from build123d import *

# Parameters (mm, degrees)
SCHIZZO1_R                   = 14
ESTRUSIONE_ESTRUSIONE1_DEPTH = 19.5
TAGLIO_ESTRUSIONE1_START     = -4
SCHIZZO2_R                   = 1
TAGLIO_ESTRUSIONE1_DEPTH     = 4
SCHIZZO3_R                   = 4.27486225
ESTRUSIONE_ESTRUSIONE2_DEPTH = 1.5
SCHIZZO4_R                   = 11.5
TAGLIO_ESTRUSIONE2_DEPTH     = 16.5
SCHIZZO5_R                   = 1.5
TAGLIO_ESTRUSIONE3_DEPTH     = 16.5
TAGLIO_ESTRUSIONE4_START     = -4
TAGLIO_ESTRUSIONE4_DEPTH     = 4
SCHIZZO7_R                   = 1.5
ESTRUSIONE_ESTRUSIONE3_DEPTH = 27.5
SCHIZZO8_R                   = 4
ESTRUSIONE_ESTRUSIONE4_DEPTH = 3
SCHIZZO9_W                   = 0.1
SCHIZZO9_H                   = 14.938811625
SMUSSO1_SIZE                 = 3.5
SMUSSO1_SIZE2                = 0.680331082
SMUSSO2_SIZE                 = 0.720279458
SMUSSO2_SIZE_2               = 3.5


with BuildPart() as part:
    # Schizzo1 → Estrusione-Estrusione1 (new body)
    with BuildSketch(Plane(origin=(0, 0, 0), x_dir=(1, 0, 0), z_dir=(0, 1, 0))):
        with Locations(Location((0, 0, 0), (0, 0, 270))):
            Circle(SCHIZZO1_R)
    extrude(amount=ESTRUSIONE_ESTRUSIONE1_DEPTH)

    # Schizzo2 → Taglio-Estrusione1 (cut)
    with BuildSketch(Plane(origin=(0, 19.5, 0), x_dir=(1, 0, 0), z_dir=(0, 1, 0)).offset(TAGLIO_ESTRUSIONE1_START)):
        with BuildLine():
            Line((-7.95445115, 11.520707743), (0, 4.27486225))
            Line((0, 4.27486225), (7.95445115, 11.520707743))
            ThreePointArc((7.95445115, 11.520707743), (0, 14), (-7.95445115, 11.520707743))
        make_face()
        with BuildLine():
            ThreePointArc((14, 0), (13.988608153, 0.564660915), (13.95445115, 1.128402898))
            Line((13.95445115, 1.128402898), (3.702139306, -2.137431125))
            Line((3.702139306, -2.137431125), (6, -12.649110641))
            ThreePointArc((6, -12.649110641), (11.832159566, -7.483314774), (14, 0))
        make_face()
        with BuildLine():
            Line((-3.702139306, -2.137431125), (-13.95445115, 1.128402898))
            ThreePointArc((-13.95445115, 1.128402898), (-12.124355653, -7), (-6, -12.649110641))
            Line((-6, -12.649110641), (-3.702139306, -2.137431125))
        make_face()
        with Locations(Location((0, -6, 0), (0, 0, 270))):
            Circle(SCHIZZO2_R)
        with Locations(Location((-5.196152423, 3, 0), (0, 0, 270))):
            Circle(SCHIZZO2_R)
        with Locations(Location((5.196152423, 3, 0), (0, 0, 270))):
            Circle(SCHIZZO2_R)
    extrude(amount=TAGLIO_ESTRUSIONE1_DEPTH, mode=Mode.SUBTRACT)

    # Schizzo3 → Estrusione-Estrusione2 (add)
    with BuildSketch(Plane(origin=(0, 19.5, 0), x_dir=(1, 0, 0), z_dir=(0, 1, 0))):
        with Locations(Location((0, 0, 0), (0, 0, 90))):
            Circle(SCHIZZO3_R)
    extrude(amount=ESTRUSIONE_ESTRUSIONE2_DEPTH)

    # Schizzo4 → Taglio-Estrusione2 (cut)
    with BuildSketch(Plane.XZ):
        with Locations(Location((0, 0, 0), (0, 0, 270))):
            Circle(SCHIZZO4_R)
    extrude(amount=-TAGLIO_ESTRUSIONE2_DEPTH, mode=Mode.SUBTRACT)

    # Schizzo5 → Taglio-Estrusione3 (cut)
    with BuildSketch(Plane(origin=(0, 21, 0), x_dir=(1, 0, 0), z_dir=(0, 1, 0))):
        with Locations(Location((0, 0, 0), (0, 0, 270))):
            Circle(SCHIZZO5_R)
    extrude(amount=-TAGLIO_ESTRUSIONE3_DEPTH, mode=Mode.SUBTRACT)

    # Schizzo6 → Taglio-Estrusione4 (cut)
    with BuildSketch(Plane(origin=(0, 19.5, 0), x_dir=(1, 0, 0), z_dir=(0, 1, 0)).offset(TAGLIO_ESTRUSIONE4_START)):
        with BuildLine():
            Line((1.5, -13.919410907), (1.5, -11.5))
            ThreePointArc((1.5, -11.5), (0, -10), (-1.5, -11.5))
            Line((-1.5, -11.5), (-1.5, -13.919410907))
            ThreePointArc((-1.5, -13.919410907), (0, -14), (1.5, -13.919410907))
        make_face()
        with BuildLine():
            ThreePointArc((9.209292144, 7.049038106), (8.660254038, 5), (10.709292144, 4.450961894))
            Line((10.709292144, 4.450961894), (12.804563451, 5.660667348))
            ThreePointArc((12.804563451, 5.660667348), (12.124355653, 7), (11.304563451, 8.258743559))
            Line((11.304563451, 8.258743559), (9.209292144, 7.049038106))
        make_face()
        with BuildLine():
            ThreePointArc((-10.709292144, 4.450961894), (-8.660254038, 5), (-9.209292144, 7.049038106))
            Line((-9.209292144, 7.049038106), (-11.304563451, 8.258743559))
            ThreePointArc((-11.304563451, 8.258743559), (-12.124355653, 7), (-12.804563451, 5.660667348))
            Line((-12.804563451, 5.660667348), (-10.709292144, 4.450961894))
        make_face()
    extrude(amount=TAGLIO_ESTRUSIONE4_DEPTH, mode=Mode.SUBTRACT)

    # Schizzo7 → Estrusione-Estrusione3 (add)
    with BuildSketch(Plane(origin=(0, 21, 0), x_dir=(1, 0, 0), z_dir=(0, 1, 0))):
        with Locations(Location((0, 0, 0), (0, 0, 270))):
            Circle(SCHIZZO7_R)
    extrude(amount=-ESTRUSIONE_ESTRUSIONE3_DEPTH)

    # Schizzo8 → Estrusione-Estrusione4 (add)
    with BuildSketch(Plane.XZ.offset(-16.5)):
        with Locations(Location((0, 0, 0), (0, 0, 270))):
            Circle(SCHIZZO8_R)
    extrude(amount=ESTRUSIONE_ESTRUSIONE4_DEPTH)

    # Schizzo9 → Rivoluzione1 (revolve)
    with BuildSketch(Plane.XY, mode=Mode.PRIVATE) as rivoluzione1_sk:
        with Locations((-14.05, 7.469405813)):
            Rectangle(SCHIZZO9_W, SCHIZZO9_H)
    revolve(rivoluzione1_sk.sketch.rotate(Axis((0, -6.5, 0), (0, 1, 0)), 270), axis=Axis((0, -6.5, 0), (0, 1, 0)))

    # Smusso1
    smusso1_edges = [part.edges().sort_by_distance(p)[0] for p in [
        (9.766653134, 19.5, -10.030577579),
        (-13.570061565, 19.5, -3.442880935),
        (13.570061565, 19.5, -3.442880935),
        (-3.803408431, 19.5, 13.473458513),
        (-9.766653134, 19.5, -10.030577579),
        (3.803408431, 19.5, 13.473458513),
    ]]
    smusso1_side = [part.faces().sort_by_distance(p)[0] for p in [
        (0, 17.219405813, -14),
    ]]
    chamfer(smusso1_edges, length=SMUSSO1_SIZE, length2=SMUSSO1_SIZE2, reference=smusso1_side[0])

    # Smusso2
    # the kernel refuses this chamfer: 3.5, 0.720279458 mm, written as the material it takes off along each edge
    with BuildSketch(Plane(origin=(0, 19.5, 0), x_dir=(-0.4593857913267627, 0, -0.8882368460760249), z_dir=(0.8882368460760249, 0, -0.4593857913267627))) as smusso2_piece_1:
        Polygon((13.319668918 + SMUSSO2_SIZE * 0.190808995258, -SMUSSO2_SIZE * 0.981627182836), (13.319668918 - SMUSSO2_SIZE_2, 0), (13.319668918, 0), align=None)
    revolve(axis=Axis((0, 19.5, 0), (0, 1, 0)), revolution_arc=97.827137871, mode=Mode.SUBTRACT)
    with BuildSketch(Plane(origin=(0, 19.5, 0), x_dir=(-0.5395427776158211, 0, 0.8419581884646081), z_dir=(-0.8419581884646081, 0, -0.5395427776158211))) as smusso2_piece_2:
        Polygon((13.319668918 + SMUSSO2_SIZE * 0.190808995258, -SMUSSO2_SIZE * 0.981627182836), (13.319668918 - SMUSSO2_SIZE_2, 0), (13.319668918, 0), align=None)
    revolve(axis=Axis((0, 19.5, 0), (0, 1, 0)), revolution_arc=97.827137871, mode=Mode.SUBTRACT)
    with BuildSketch(Plane(origin=(0, 19.5, 0), x_dir=(0.8174001702166583, 0, 0.5760702749923641), z_dir=(-0.5760702749923641, 0, 0.8174001702166583))) as smusso2_piece_3:
        Polygon((13.319668918 + SMUSSO2_SIZE * 0.190808995258, -SMUSSO2_SIZE * 0.981627182836), (13.319668918 - SMUSSO2_SIZE_2, 0), (13.319668918, 0), align=None)
    revolve(axis=Axis((0, 19.5, 0), (0, 1, 0)), revolution_arc=97.827137871, mode=Mode.SUBTRACT)


solid = part.part
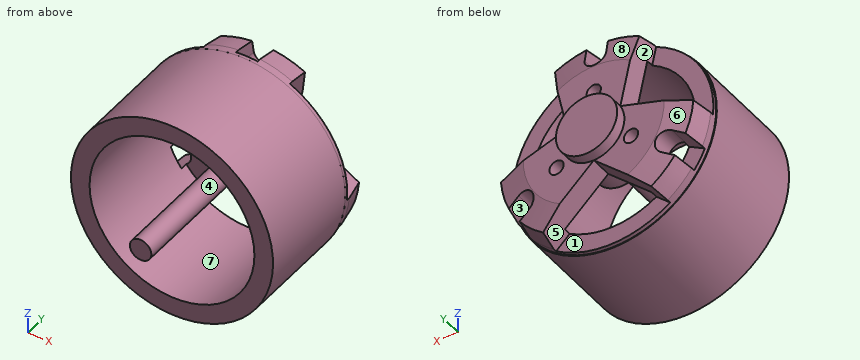
CAD build for the part. Positions are in the model's coordinates, mm. Face numbers are marked on the shaded views. A direction names the side the tool comes from. Round coordinates to 2 decimals unless told otherwise and drop trailing zeros. Order: outer loops, then holes, each group sorted by start corner. A loop starts at its lowest first (then second) coordinate and runs counter-clockwise, first axis right, second up. Notation, with made-up numbers: (76, 85) - (110, 85) arc R37 ccw to (110, 121) - close; hole circle Ø5 at (50.25, -12). An arc over 180 degrees is marked (long way). Return JSON: item names as keys, results as strings.
(1) Cut at A-A (z = 6). Give the cut face in (x, y).
Answer key:
{"outline": "(-12.76, 0) - (-9.81, 0) - (-9.81, 15.5) - (-12.65, 15.5) - (-12.65, 14.94) - (-12.76, 14.94) - close; (-4.55, 16.5) - (-1, 16.5) - (-1, 19.5) - (-4.55, 19.5) - close; (1, 16.5) - (4.55, 16.5) - (4.55, 19.5) - (1, 19.5) - close; (9.81, 0) - (12.76, 0) - (12.76, 14.94) - (12.65, 14.94) - (12.65, 15.5) - (9.81, 15.5) - close"}
(2) Cut at C-C (y = 17.5). Give the cut face in (x, z), then the cut area to 3 significant figures.
Answer key:
{"outline": "(-13.67, -1.04) arc R13.71 ccw to (-12.55, -5.51) - (-10.71, -4.45) arc R1.5 cw to (-9.21, -7.05) - (-11.05, -8.11) arc R13.71 ccw to (-7.73, -11.32) - (0, -4.27) - (7.73, -11.32) arc R13.71 ccw to (11.05, -8.11) - (9.21, -7.05) arc R1.5 cw to (10.71, -4.45) - (12.55, -5.51) arc R13.71 ccw to (13.67, -1.04) - (3.7, 2.14) - (5.94, 12.36) arc R13.71 ccw to (1.5, 13.63) - (1.5, 11.5) arc R1.5 cw to (-1.5, 11.5) - (-1.5, 13.63) arc R13.71 ccw to (-5.94, 12.36) - (-3.7, 2.14) - close; hole circle Ø2 at (-5.2, -3); hole circle Ø2 at (0, 6); hole circle Ø2 at (5.2, -3)", "area": "312 mm^2"}
(3) Tool access for the marked faces 1, 2, 3 and 4: list every direction of +Z, -Z, +X, -X, +Y, -Y with a clear straight run to the whole face (end or side of a thin tool).
Answer key:
{"face 1": "-Z, +Y", "face 2": "-X, +Y", "face 3": "+Y", "face 4": "-Y"}
(4) Pin check, flat tips, straight feed: pin 1 Ø3 at (y, z) = (15.5, -0.5) entering from +X; pin 2 Ø3 at (x, y) = (-8.5, 3.5) entering from -Z; pin 3 Ø2.5 at (y, z) = (18, 13.5) entering from +X; pin 4 Ø2.5 at (x, z) = (-5.2, -3) entering from -Y. Stop position of each tip, or through.
Answer key:
{"pin 1": "stops at x = 14.1", "pin 2": "stops at z = -12.24", "pin 3": "stops at x = 5.94", "pin 4": "stops at y = 16.5"}
(5) Wall check: probe 1 along X at (y, z) = (17.8, -3); probe 2 along Z at (x, y) = (1.25, 8.75); probe 3 along X at (y, z) = (17.4, -3). Give the ranges that are in metal, low to high. Write a range as from..to.
Answer key:
{"probe 1": "x = -13.32..-6.2, -4.2..4.2, 6.2..13.32", "probe 2": "z = -14.04..-11.43, -0.83..0.83, 11.43..14.04", "probe 3": "x = -13.4..-6.2, -4.2..4.2, 6.2..13.4"}
(6) Cut at D-D (y = -3.5). Give the cut face in (x, z), then the cut area to 3 significant figures.
Answer key:
{"outline": "circle Ø3 at (0, 0)", "area": "7.07 mm^2"}
(7) Cut at B-B (y = 8.75). Give the cut face in (x, z), then the cut area to 3 significant figures.
Answer key:
{"outline": "circle Ø28.2 at (0, 0); circle Ø3 at (0, 0); hole circle Ø23 at (0, 0)", "area": "216 mm^2"}
(8) Pull direction X, two halves, no side cores. Call the marked faces 5, 6, 7 and 8: +X half, -X half, draft (parallel to the pull), parting line (faces both ways), or undercut.
Answer key:
{"face 5": "undercut", "face 6": "-X half", "face 7": "undercut", "face 8": "parting line"}
